Read the model definition and answer for the solid it produces. Units are mm, in the model's axes. A direction names the side the tool comes from. Give positions to 0.01 mm unless a question says otherwise; leave off trailing zeros. Order: outer loops, then holes, each group sorted by start corner. A loop starts at its lowest first (then second) coordinate and runs counter-clockwise, first axis right, second up. Notation, with made-up numbers: (29.5, -37.5) -> (34.5, -37.5) arc R25 cw to (34.5, -6.5) -> close; hole circle Ø10 at (41, 7.25). An arc over 180 degrees is marked (long way). Answer as CSV lines item,"result". Start each with the question number.
1) Flat-ended cylindrical pins translate along their axes: pin 1 Ø2 at (x, y) = (98, 25) entering from -Z; pin 2 Ø8 at (y, z) = (29.5, 6.5) entering from +X; pin 3 Ø5 at (y, z) = (-18.5, -17) entering from -X; pin 4 Ø4 at (y, z) = (0, -0.5) entering from -X. Find the tip coordinate at first contact, or state that the pin passes through.
2) Find section D-D (z = 4.5). Determine the outline of the cut face in (x, y), and give its area (3 significant figures).
3) Find section B-B (x = 0). Determine the outline of the cut face in (y, z).
4) The mould has two halves that part along X. Classify faces 1 (the face through (56.205, 3.135, 5.03)), 2 (the face through (10.16, -26, 5)), 3 (the face through (14, -15, -23.368)): +X half, -X half, draft (parallel to the pull), parting line (faces both ways), or undercut.
5) Find section C-C (y = 32). Determine the outline of the cut face in (x, z), and give its area (3 significant figures).
6) For faces 4 (the face through (10.16, 27, 5)), 5 (the face through (0.08, -37.72, 9.26)), 6 (the face through (6.604, 0, 4)), 7 (the face through (99, 23, -22.86)), 8 (the face through (101.328, -3.883, -11.59)), determine the directions among +Z, -Z, +X, -X, +Y, -Y from which every point of the face is accessible in a straight line to the end or side of a thin tool.
7) Straight lines are drawn through the part: L1, parallel to X at y = -7, z = 7; L2, parallel to X at y = -25.5, z = 1; L3, parallel to Z at x = 11, y = -5. For each, find the intervals that lie inside material, in ascending order. Write a range as from..to.
8) Find section A-A (z = -12). Determine the outline of the cut face in (x, y), and give its area (3 significant figures).
```python
from build123d import *

# Parameters (mm, degrees)
SKETCH1_R           = 10.16
SKETCH1_W           = 20.32
SKETCH1_H           = 68.58
BOSS_EXTRUDE1_DEPTH = 10.16
SKETCH2_R           = 6.604
SKETCH2_W           = 13.208
SKETCH2_H           = 68.58
CUT_EXTRUDE1_DEPTH  = 47.714598361
BOSS_EXTRUDE2_DEPTH = 10.16
SKETCH4_W           = 33.528
SKETCH4_H           = 38.1
BOSS_EXTRUDE3_DEPTH = 6.35
SKETCH5_W           = 23.368
SKETCH5_H           = 25.4
CUT_EXTRUDE2_DEPTH  = 102.646087633
SKETCH6_W           = 33.02
SKETCH6_H           = 38.1
BOSS_EXTRUDE4_DEPTH = 6.35
BOSS_EXTRUDE5_REACH = 110.063
SKETCH7_W           = 10.16
SKETCH7_H           = 14.989497654
SKETCH8_W           = 22.86
SKETCH8_H           = 22.86
CUT_EXTRUDE3_DEPTH  = 122.879251037
SKETCH9_R           = 3.175
BOSS_EXTRUDE6_DEPTH = 6.35
SKETCH10_R          = 3.175
BOSS_EXTRUDE7_DEPTH = 6.35
SKETCH13_R          = 2.286
CUT_EXTRUDE4_DEPTH  = 81.28
BOSS_EXTRUDE8_START = -1.778
BOSS_EXTRUDE8_DEPTH = 1.778


with BuildPart() as part:
    # Sketch1 → Boss-Extrude1 (new body)
    with BuildSketch(Plane.XY):
        with Locations((0, 34.29)):
            Circle(SKETCH1_R)
        with Locations((0, -34.29)):
            Circle(SKETCH1_R)
        Rectangle(SKETCH1_W, SKETCH1_H)
    extrude(amount=BOSS_EXTRUDE1_DEPTH)

    # Sketch2 → Cut-Extrude1 (cut, through all)
    with BuildSketch(Plane.XY.offset(10.16)):
        with Locations((0, 34.29)):
            Circle(SKETCH2_R)
        with Locations((0, -34.29)):
            Circle(SKETCH2_R)
        Rectangle(SKETCH2_W, SKETCH2_H)
    extrude(amount=-CUT_EXTRUDE1_DEPTH, mode=Mode.SUBTRACT)

    # Sketch3 → Boss-Extrude2 (add)
    with BuildSketch(Plane(origin=(0, 0, 0), x_dir=(-1, 0, 0), z_dir=(0, 0, -1))):
        Polygon((-9.606561034, 3.138708349), (-103.22893876, 11.329605052), (-103.782377727, 5.003768719), (-10.16, -3.187127984), align=None)
    extrude(amount=-BOSS_EXTRUDE2_DEPTH)

    # Sketch4 → Boss-Extrude3 (add)
    with BuildSketch(Plane(origin=(-103.08224956, 1291.177707373, 0), x_dir=(0, 0, -1), z_dir=(-0.9961946980917459, -0.08715574274765499, 0))):
        with Locations((6.604, 1295.248596403)):
            Rectangle(SKETCH4_W, SKETCH4_H)
    extrude(amount=-BOSS_EXTRUDE3_DEPTH)

    # Sketch5 → Cut-Extrude2 (cut, through all)
    with BuildSketch(Plane(origin=(16.131940235, 1.411361891, 0), x_dir=(0, 0, 1), z_dir=(0.9961946980917458, 0.08715574274765524, 0))):
        with Locations((-11.684, 0)):
            Rectangle(SKETCH5_W, SKETCH5_H)
    extrude(amount=-CUT_EXTRUDE2_DEPTH, mode=Mode.SUBTRACT)

    # Sketch6 → Boss-Extrude4 (add)
    with BuildSketch(Plane(origin=(103.428481629, 9.048819628, 0), x_dir=(0, 0, -1), z_dir=(0.9961946980917468, 0.08715574274764347, 0))):
        with Locations((6.35, 0)):
            Rectangle(SKETCH6_W, SKETCH6_H)
    extrude(amount=-BOSS_EXTRUDE4_DEPTH)

    # Sketch7 → Boss-Extrude5 (add, up to next)
    with BuildSketch(Plane(origin=(9.806103902, 0.857922925, 0), x_dir=(0, 0, 1), z_dir=(-0.9961946980917458, -0.08715574274765528, 0)), mode=Mode.PRIVATE) as boss_extrude5_sk1:
        with Locations((5.08, -11.555251173)):
            Rectangle(SKETCH7_W, SKETCH7_H)
    boss_extrude5_tool1 = extrude(boss_extrude5_sk1.sketch, amount=BOSS_EXTRUDE5_REACH, mode=Mode.PRIVATE) - part.part
    add(boss_extrude5_tool1.solids().sort_by_distance((10.81321, -10.653357, 5.08))[0])

    # Sketch8 → Cut-Extrude3 (cut, through all)
    with BuildSketch(Plane(origin=(97.102645296, 8.495380662, 0), x_dir=(0, 0, 1), z_dir=(-0.9961946980917469, -0.08715574274764348, 0))):
        with Locations((-11.43, -1.27)):
            Rectangle(SKETCH8_W, SKETCH8_H)
    extrude(amount=-CUT_EXTRUDE3_DEPTH, mode=Mode.SUBTRACT)

    # Sketch9 → Boss-Extrude6 (add)
    with BuildSketch(Plane(origin=(9.806103902, 0.857922925, 0), x_dir=(0, 0, 1), z_dir=(-0.9961946980917459, -0.0871557427476546, 0))):
        with Locations((-20.193, 12.7)):
            Circle(SKETCH9_R)
    extrude(amount=-BOSS_EXTRUDE6_DEPTH)

    # Sketch10 → Boss-Extrude7 (add)
    with BuildSketch(Plane(origin=(97.102645296, 8.495380662, 0), x_dir=(0, 0, 1), z_dir=(-0.9961946980917469, -0.08715574274764348, 0))):
        with Locations((-19.685, 10.16)):
            Circle(SKETCH10_R)
    extrude(amount=-BOSS_EXTRUDE7_DEPTH)

    # Sketch13 → Cut-Extrude4 (cut)
    with BuildSketch(Plane(origin=(16.131940235, 1.411361891, 0), x_dir=(0, 0, -1), z_dir=(0.9961946980917459, 0.0871557427476546, 0))):
        with Locations((-5.08, -4.060502346)):
            Circle(SKETCH13_R)
    extrude(amount=CUT_EXTRUDE4_DEPTH, mode=Mode.SUBTRACT)

    # Sketch14 → Boss-Extrude8 (add)
    with BuildSketch(Plane.XY.offset(10.16).offset(BOSS_EXTRUDE8_START)):
        with BuildLine():
            Line((-10.16, -34.29), (-10.16, 34.29))
            ThreePointArc((-10.16, 34.29), (0, 44.45), (10.16, 34.29))
            Line((10.16, 34.29), (10.16, -34.29))
            ThreePointArc((10.16, -34.29), (0, -44.45), (-10.16, -34.29))
        make_face()
        with BuildLine():
            Line((-3.429, -34.29), (-3.429, 34.29))
            ThreePointArc((-3.429, 34.29), (0, 37.719), (3.429, 34.29))
            Line((3.429, 34.29), (3.429, -34.29))
            ThreePointArc((3.429, -34.29), (0, -37.719), (-3.429, -34.29))
        make_face(mode=Mode.SUBTRACT)
    extrude(amount=BOSS_EXTRUDE8_DEPTH)


solid = part.part
```
Findings below:
1,pin 1,"z = -22.86"
1,pin 2,"x = 101.99"
1,pin 3,"x = 11.28"
1,pin 4,"x = -10.16"
2,outline,"(-10.16, -34.29) arc R10.16 ccw to (10.16, -34.29) -> (10.16, -18.23) -> (17.79, -17.57) -> (16.29, -0.43) -> (97.26, 6.65) -> (98.76, -10.48) -> (105.09, -9.93) -> (101.77, 28.03) -> (95.44, 27.47) -> (96.9, 10.78) -> (15.93, 3.69) -> (14.47, 20.39) -> (10.16, 20.01) -> (10.16, 34.29) arc R10.16 ccw to (-10.16, 34.29) -> close; hole (-6.6, -34.29) arc R6.6 ccw to (6.6, -34.29) -> (6.6, 34.29) arc R6.6 ccw to (-6.6, 34.29) -> close"
2,area,"1,480 mm²"
3,outline,"(-44.45, 0) -> (-40.89, 0) -> (-40.89, 8.38) -> (-37.72, 8.38) -> (-37.72, 10.16) -> (-44.45, 10.16) -> close; (37.72, 8.38) -> (40.89, 8.38) -> (40.89, 0) -> (44.45, 0) -> (44.45, 10.16) -> (37.72, 10.16) -> close"
4,face 1,"undercut"
4,face 2,"+X half"
4,face 3,"draft"
5,outline,"(-10.16, 0) -> (-6.6, 0) -> (-6.6, 8.38) -> (-3.43, 8.38) -> (-3.43, 10.16) -> (-10.16, 10.16) -> close; (3.43, 8.38) -> (6.6, 8.38) -> (6.6, 0) -> (10.16, 0) -> (10.16, 10.16) -> (3.43, 10.16) -> close"
5,area,"83.5 mm²"
6,face 4,"+Z, -Z, +Y"
6,face 5,"+Z, -Z"
6,face 6,"-Z"
6,face 7,"-Z, +X, +Y, -Y"
6,face 8,"-Z, -X"
7,L1,"-10.16..-6.6, 6.6..16.87, 98.46..104.83"
7,L2,"-10.16..-6.6, 6.6..10.16"
7,L3,"0..10.16"
8,outline,"(8.15, 19.84) -> (8.7, 13.51) -> (15.03, 14.06) -> (14.47, 20.39) -> close; (10.91, -11.79) -> (11.47, -18.12) -> (17.79, -17.57) -> (17.24, -11.24) -> close; (95.44, 27.47) -> (96.22, 18.62) -> (102.54, 19.17) -> (101.77, 28.03) -> close; (98.21, -4.16) -> (98.76, -10.48) -> (105.09, -9.93) -> (104.54, -3.6) -> close"
8,area,"177 mm²"
